```python
from build123d import *

# Parameters (mm, degrees)
F0_W     = 25
F0_H     = 30
F1_DEPTH = 2
F2_R     = 1.5
F3_DEPTH = 2.001
F4_W     = 1
F4_H     = 6.1
F5_DEPTH = 0.7
F6_SIZE  = 10
F7_R     = 7


with BuildPart() as f1:
    # F0 (on Top) → F1 (new body)
    with BuildSketch(Plane.XY):
        Rectangle(F0_W, F0_H)
    extrude(amount=F1_DEPTH)

    # F2 (on face) → F3 (cut, through all)
    with BuildSketch(Plane.XY.offset(2)):
        with Locations((-2, -12)):
            Circle(F2_R)
        with Locations((4.5, -1.5)):
            Circle(F2_R)
        with Locations((4.5, 8.5)):
            Circle(F2_R)
    extrude(amount=-F3_DEPTH, mode=Mode.SUBTRACT)

    # F4 (on face) → F5 (cut)
    with BuildSketch(Plane.XY.offset(2)):
        with Locations((11.6, -6.95)):
            Rectangle(F4_W, F4_H)
        with Locations((9.6, -6.95)):
            Rectangle(F4_W, F4_H)
        with Locations((7.6, -6.95)):
            Rectangle(F4_W, F4_H)
        with Locations((5.6, -6.95)):
            Rectangle(F4_W, F4_H)
        with Locations((3.6, -6.95)):
            Rectangle(F4_W, F4_H)
        with Locations((1.6, -6.95)):
            Rectangle(F4_W, F4_H)
        with Locations((-0.4, -6.95)):
            Rectangle(F4_W, F4_H)
        with Locations((-2.4, -6.95)):
            Rectangle(F4_W, F4_H)
        with Locations((-4.4, -6.95)):
            Rectangle(F4_W, F4_H)
        with Locations((-6.4, -6.95)):
            Rectangle(F4_W, F4_H)
        with Locations((-8.4, -6.95)):
            Rectangle(F4_W, F4_H)
        with Locations((-10.4, -6.95)):
            Rectangle(F4_W, F4_H)
        with Locations((-12.4, -6.95)):
            Rectangle(F4_W, F4_H)
    extrude(amount=-F5_DEPTH, mode=Mode.SUBTRACT)

    # F6
    f6_edges = [f1.edges().sort_by_distance(p)[0] for p in [
        (-12.5, 15, 1),
    ]]
    chamfer(f6_edges, length=F6_SIZE)

    # F7
    f7_edges = [f1.edges().sort_by_distance(p)[0] for p in [
        (-12.5, 5, 1),
        (-2.5, 15, 1),
        (12.5, 15, 1),
    ]]
    fillet(f7_edges, radius=F7_R)


solid = f1.part
```
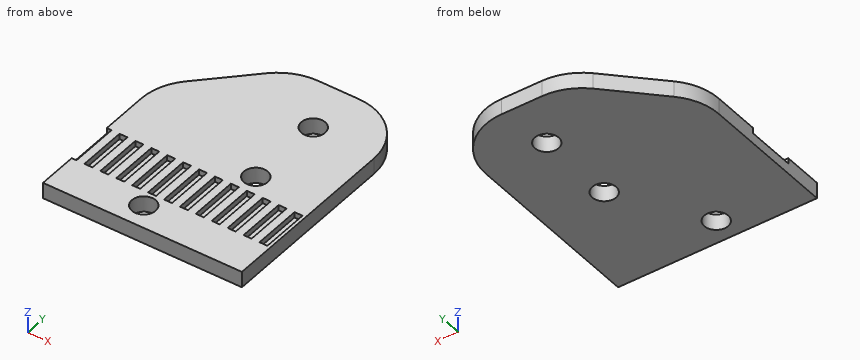
Could you check a few things on this model? Use its own coordinates, in mm. Round coordinates to 2 decimals unless told otherwise and drop trailing zeros. Loops run counter-clockwise (first coordinate to the right, second up) from the corner with the lowest first, then second, coordinate; pieces in that order, holes last. Notation, with made-up numbers: (11, 50) - (31, 50) arc R30 cw to (31, 84) - close; hole circle Ø6 at (-20.75, 27.25). An arc over 180 degrees is marked (long way). Answer as CSV lines item,"result".
1. Please list where these lines run through material, in increasing order: line 1 along Y through (x, z) = (4.5, 1.5); line 2 along Y through (x, z) = (3.25, 1.85); line 3 along Z through (x, y) = (-2.75, -4.5). Write a range as [from, to].
Filled in:
line 1,"y = [-15, -3], [0, 7], [10, 15]"
line 2,"y = [-15, -10], [-3.9, -2.33], [-0.67, 7.67], [9.33, 15]"
line 3,"z = [0, 1.3]"
2. I want a section at D-D on y = 8.5. List the corners of the cut face in (x, z) for me, then the cut area to 3 significant figures.
Filled in:
outline,"(-9, 0) - (3, 0) - (3, 2) - (-9, 2) - close; (6, 0) - (12.48, 0) - (12.48, 2) - (6, 2) - close"
area,"37.0 mm^2"
3. I want a section at A-A on y = -1.5. List the corners of the cut face in (x, z) for me.
Filled in:
outline,"(-12.5, 0) - (3, 0) - (3, 2) - (-12.5, 2) - close; (6, 0) - (12.5, 0) - (12.5, 2) - (6, 2) - close"
4. I want a section at C-C on x = -8.5. List the corners of the cut face in (y, z) for me.
Filled in:
outline,"(-15, 0) - (9, 0) - (9, 2) - (-3.9, 2) - (-3.9, 1.3) - (-10, 1.3) - (-10, 2) - (-15, 2) - close"
5. I want a section at B-B on z = 0.65. List the corners of the cut face in (x, y) for me.
Filled in:
outline,"(-12.5, -15) - (12.5, -15) - (12.5, 8) arc R7 ccw to (5.5, 15) - (0.4, 15) arc R7 ccw to (-4.55, 12.95) - (-10.45, 7.05) arc R7 ccw to (-12.5, 2.1) - close; hole circle Ø3 at (-2, -12); hole circle Ø3 at (4.5, -1.5); hole circle Ø3 at (4.5, 8.5)"
